Could you check a few things on this model? Use its own coordinates, in mm. Coordinates: 2 decimals unless noted, no trailing zeros. Loops run counter-clockwise (first coordinate to the right, second up) from the corner with the lowest first, then second, coordinate; pieces in that order, holes last. Notation, with made-up numbers: (73.25, -24) - (93.25, -24) arc R30 ccw to (93.25, 9) - close; hole circle Ø9 at (84, 79.5). An arc over 180 degrees is marked (long way). One line per item, written item: value. Start each with the question number.
(1) I'm going to push flat-ended pins straight in: P1, Ø2, axis at x = -120.5, z = 3, coming from the -Y side; P2, Ø1.5, axis at x = -78.5, y = 12.5, coming from the -Z side; P3, Ø3.5, axis at x = -36, z = 1.5, coming from the -Y side; P4, Ø2.5, axis at x = -160.43, y = -41.87, coming from the -Z side. Where does each tip first touch, or does it pass through?
(2) If I drill on line 1 along Y through (x, z) = (-158, 2.5); line 2 along Y through (x, z) = (-161, 4.25); line 3 along Y through (x, z) = (-144, 1.75), over which ranges is the centre line in solid material (lowest first)? Write a range as from..to.
(3) If we section it at B-B on x = -134: Write out the boundary of the cut face in (y, z), then the cut area to 3 significant figures.
(4) If we section it at C-C on x = -38: Count the separate pieces of the cut face and the enclosed holes in it, then the cut area to 3 significant figures.
(5) If we section it at A-A on z = -1: Write out the boundary of the cut face in (x, y), then the cut area to 3 significant figures.
```python
from build123d import *

# Parameters (mm, degrees)
F0_R     = 1.5
F0_R_2   = 4.064442
F0_W     = 17.869964
F0_H     = 3
F1_DEPTH = 4.5
F2_W     = 10.996489
F2_H     = 3.251471
F3_DEPTH = 2
F4_R     = 5.902111
F5_DEPTH = 2
F7_DEPTH = 25


with BuildPart() as f1:
    # F0 (on Top) → F1 (new body)
    with BuildSketch(Plane.XY):
        with BuildLine():
            ThreePointArc((0, 42.5), (-1.464466, 46.035534), (-5, 47.5))
            Line((-5, 47.5), (-22.221084, 47.5))
            ThreePointArc((-22.221084, 47.5), (-23.18507, 47.406193), (-24.112885, 47.128292))
            Line((-24.112885, 47.128292), (-53.784762, 35))
            Line((-53.784762, 35), (-94.883973, 35))
            ThreePointArc((-94.883973, 35), (-97.317732, 34.367701), (-99.135947, 32.630726))
            ThreePointArc((-99.135947, 32.630726), (-115.303652, 25.021468), (-128.810321, 36.720415))
            ThreePointArc((-128.810321, 36.720415), (-129.96409, 38.753765), (-131.916134, 40.040317))
            Line((-131.916134, 40.040317), (-152.559489, 47.5))
            Line((-152.559489, 47.5), (-165, 47.5))
            ThreePointArc((-165, 47.5), (-168.535534, 46.035534), (-170, 42.5))
            Line((-170, 42.5), (-170, 35))
            Line((-170, 35), (-170, 0))
            Line((-170, 0), (-170, -35))
            Line((-170, -35), (-170, -42.5))
            ThreePointArc((-170, -42.5), (-168.535534, -46.035534), (-165, -47.5))
            Line((-165, -47.5), (-152.559489, -47.5))
            Line((-152.559489, -47.5), (-131.916134, -40.040317))
            ThreePointArc((-131.916134, -40.040317), (-129.96409, -38.753765), (-128.810321, -36.720415))
            ThreePointArc((-128.810321, -36.720415), (-115.303652, -25.021468), (-99.135947, -32.630726))
            ThreePointArc((-99.135947, -32.630726), (-97.317732, -34.367701), (-94.883973, -35))
            Line((-94.883973, -35), (-53.784762, -35))
            Line((-53.784762, -35), (-24.112885, -47.128292))
            ThreePointArc((-24.112885, -47.128292), (-23.18507, -47.406193), (-22.221084, -47.5))
            Line((-22.221084, -47.5), (-5, -47.5))
            ThreePointArc((-5, -47.5), (-1.464466, -46.035534), (0, -42.5))
            Line((0, -42.5), (0, -35))
            Line((0, -35), (0, 0))
            Line((0, 0), (0, 35))
            Line((0, 35), (0, 42.5))
        make_face()
        with Locations((-160.42681, -41.874927)):
            Circle(F0_R, mode=Mode.SUBTRACT)
        with Locations((-165.596247, -31.161871)):
            Circle(F0_R, mode=Mode.SUBTRACT)
        with Locations((-157.563224, -27.604574)):
            Circle(F0_R_2, mode=Mode.SUBTRACT)
        with Locations((-94.883973, -30)):
            Circle(F0_R, mode=Mode.SUBTRACT)
        with BuildLine():
            Line((-155.63046, -13.178692), (-144.869025, -2.417256))
            ThreePointArc((-144.869025, -2.417256), (-142.747705, -2.417256), (-142.747705, -4.538577))
            Line((-142.747705, -4.538577), (-153.50914, -15.300012))
            ThreePointArc((-153.50914, -15.300012), (-155.63046, -15.300012), (-155.63046, -13.178692))
        make_face(mode=Mode.SUBTRACT)
        with BuildLine():
            Line((-126.950468, -15.501301), (-137.913192, -4.538577))
            ThreePointArc((-137.913192, -4.538577), (-137.913192, -2.417256), (-135.791872, -2.417256))
            Line((-135.791872, -2.417256), (-124.829148, -13.37998))
            ThreePointArc((-124.829148, -13.37998), (-124.829148, -15.501301), (-126.950468, -15.501301))
        make_face(mode=Mode.SUBTRACT)
        with Locations((-97.036146, -19.152308)):
            Circle(F0_R_2, mode=Mode.SUBTRACT)
        with Locations((-11.601751, -41.25)):
            Circle(F0_R, mode=Mode.SUBTRACT)
        with Locations((-37.462216, -31.5)):
            Rectangle(F0_W, F0_H, mode=Mode.SUBTRACT)
        with Locations((-3.568025, -34.615397)):
            Circle(F0_R, mode=Mode.SUBTRACT)
        with BuildLine():
            ThreePointArc((-155.63046, 13.178692), (-155.63046, 15.300012), (-153.50914, 15.300012))
            Line((-153.50914, 15.300012), (-142.747705, 4.538577))
            ThreePointArc((-142.747705, 4.538577), (-142.747705, 2.417256), (-144.869025, 2.417256))
            Line((-144.869025, 2.417256), (-155.63046, 13.178692))
        make_face(mode=Mode.SUBTRACT)
        with BuildLine():
            ThreePointArc((-135.791872, 2.417256), (-137.913192, 2.417256), (-137.913192, 4.538577))
            Line((-137.913192, 4.538577), (-126.950468, 15.501301))
            ThreePointArc((-126.950468, 15.501301), (-124.829148, 15.501301), (-124.829148, 13.37998))
            Line((-124.829148, 13.37998), (-135.791872, 2.417256))
        make_face(mode=Mode.SUBTRACT)
        with Locations((-97.036146, 19.152308)):
            Circle(F0_R_2, mode=Mode.SUBTRACT)
        with Locations((-157.563224, 27.604574)):
            Circle(F0_R_2, mode=Mode.SUBTRACT)
        with Locations((-165.596247, 31.161871)):
            Circle(F0_R, mode=Mode.SUBTRACT)
        with Locations((-160.42681, 41.874927)):
            Circle(F0_R, mode=Mode.SUBTRACT)
        with Locations((-94.883973, 30)):
            Circle(F0_R, mode=Mode.SUBTRACT)
        with Locations((-37.462216, 31.5)):
            Rectangle(F0_W, F0_H, mode=Mode.SUBTRACT)
        with Locations((-3.568025, 34.615397)):
            Circle(F0_R, mode=Mode.SUBTRACT)
        with Locations((-11.601751, 41.25)):
            Circle(F0_R, mode=Mode.SUBTRACT)
    extrude(amount=F1_DEPTH)

    # F2 (on face) → F3 (join)
    with BuildSketch(Plane(origin=(0, 0, 0), x_dir=(1, 0, 0), z_dir=(0, 0, -1))):
        with Locations((-164.501756, 34.962811)):
            Rectangle(F2_W, F2_H)
        with BuildLine():
            Line((-0.535832, 44.751933), (-7.695868, 37.591897))
            Line((-7.695868, 37.591897), (-5.774221, 35.670251))
            Line((-5.774221, 35.670251), (0, 40.31283))
            Line((0, 40.31283), (0, 42.5))
            ThreePointArc((0, 42.5), (-0.135802, 43.657402), (-0.535832, 44.751933))
        make_face()
        with BuildLine():
            Line((0, -42.5), (0, -40.31283))
            Line((0, -40.31283), (-5.774221, -35.670251))
            Line((-5.774221, -35.670251), (-7.695868, -37.591897))
            Line((-7.695868, -37.591897), (-0.535832, -44.751933))
            ThreePointArc((-0.535832, -44.751933), (-0.135802, -43.657402), (0, -42.5))
        make_face()
        with Locations((-164.501756, -34.962811)):
            Rectangle(F2_W, F2_H)
    extrude(amount=F3_DEPTH)

    # F4 (on face) → F5 (cut)
    with BuildSketch(Plane(origin=(0, 0, 0), x_dir=(1, 0, 0), z_dir=(0, 0, -1))):
        with Locations((-97.036146, 19.152308)):
            Circle(F4_R)
        with Locations((-157.563224, 27.604574)):
            Circle(F4_R)
        with Locations((-97.036146, -19.152308)):
            Circle(F4_R)
        with Locations((-157.563224, -27.604574)):
            Circle(F4_R)
    extrude(amount=-F5_DEPTH, mode=Mode.SUBTRACT)

    # F6 (on face) → F7 (cut)
    with BuildSketch(Plane(origin=(0, 0, 0), x_dir=(1, 0, 0), z_dir=(0, 0, -1))):
        with BuildLine():
            ThreePointArc((-79.22934, 23.110536), (-80.72934, 21.610536), (-79.22934, 20.110536))
            Line((-79.22934, 20.110536), (-20.462809, 20.110536))
            ThreePointArc((-20.462809, 20.110536), (-18.962809, 21.610536), (-20.462809, 23.110536))
            Line((-20.462809, 23.110536), (-79.22934, 23.110536))
        make_face()
        with BuildLine():
            Line((-20.462809, 18.110536), (-79.22934, 18.110536))
            ThreePointArc((-79.22934, 18.110536), (-80.72934, 16.610536), (-79.22934, 15.110536))
            Line((-79.22934, 15.110536), (-20.462809, 15.110536))
            ThreePointArc((-20.462809, 15.110536), (-18.962809, 16.610536), (-20.462809, 18.110536))
        make_face()
        with BuildLine():
            Line((-20.462809, 13.110536), (-79.22934, 13.110536))
            ThreePointArc((-79.22934, 13.110536), (-80.72934, 11.610536), (-79.22934, 10.110536))
            Line((-79.22934, 10.110536), (-20.462809, 10.110536))
            ThreePointArc((-20.462809, 10.110536), (-18.962809, 11.610536), (-20.462809, 13.110536))
        make_face()
        with BuildLine():
            Line((-20.462809, 8.110536), (-79.22934, 8.110536))
            ThreePointArc((-79.22934, 8.110536), (-80.72934, 6.610536), (-79.22934, 5.110536))
            Line((-79.22934, 5.110536), (-20.462809, 5.110536))
            ThreePointArc((-20.462809, 5.110536), (-18.962809, 6.610536), (-20.462809, 8.110536))
        make_face()
        with BuildLine():
            Line((-20.462809, 3.110536), (-79.22934, 3.110536))
            ThreePointArc((-79.22934, 3.110536), (-80.72934, 1.610536), (-79.22934, 0.110536))
            Line((-79.22934, 0.110536), (-20.462809, 0.110536))
            ThreePointArc((-20.462809, 0.110536), (-18.962809, 1.610536), (-20.462809, 3.110536))
        make_face()
        with BuildLine():
            Line((-20.462809, -1.889464), (-79.22934, -1.889464))
            ThreePointArc((-79.22934, -1.889464), (-80.72934, -3.389464), (-79.22934, -4.889464))
            Line((-79.22934, -4.889464), (-20.462809, -4.889464))
            ThreePointArc((-20.462809, -4.889464), (-18.962809, -3.389464), (-20.462809, -1.889464))
        make_face()
        with BuildLine():
            Line((-20.462809, -6.889464), (-79.22934, -6.889464))
            ThreePointArc((-79.22934, -6.889464), (-80.72934, -8.389464), (-79.22934, -9.889464))
            Line((-79.22934, -9.889464), (-20.462809, -9.889464))
            ThreePointArc((-20.462809, -9.889464), (-18.962809, -8.389464), (-20.462809, -6.889464))
        make_face()
        with BuildLine():
            Line((-20.462809, -11.889464), (-79.22934, -11.889464))
            ThreePointArc((-79.22934, -11.889464), (-80.72934, -13.389464), (-79.22934, -14.889464))
            Line((-79.22934, -14.889464), (-20.462809, -14.889464))
            ThreePointArc((-20.462809, -14.889464), (-18.962809, -13.389464), (-20.462809, -11.889464))
        make_face()
        with BuildLine():
            Line((-20.462809, -16.889464), (-79.22934, -16.889464))
            ThreePointArc((-79.22934, -16.889464), (-80.72934, -18.389464), (-79.22934, -19.889464))
            Line((-79.22934, -19.889464), (-20.462809, -19.889464))
            ThreePointArc((-20.462809, -19.889464), (-18.962809, -18.389464), (-20.462809, -16.889464))
        make_face()
        with BuildLine():
            Line((-20.462809, -21.889464), (-79.22934, -21.889464))
            ThreePointArc((-79.22934, -21.889464), (-80.72934, -23.389464), (-79.22934, -24.889464))
            Line((-79.22934, -24.889464), (-20.462809, -24.889464))
            ThreePointArc((-20.462809, -24.889464), (-18.962809, -23.389464), (-20.462809, -21.889464))
        make_face()
    extrude(amount=-F7_DEPTH, mode=Mode.SUBTRACT)


solid = f1.part
```
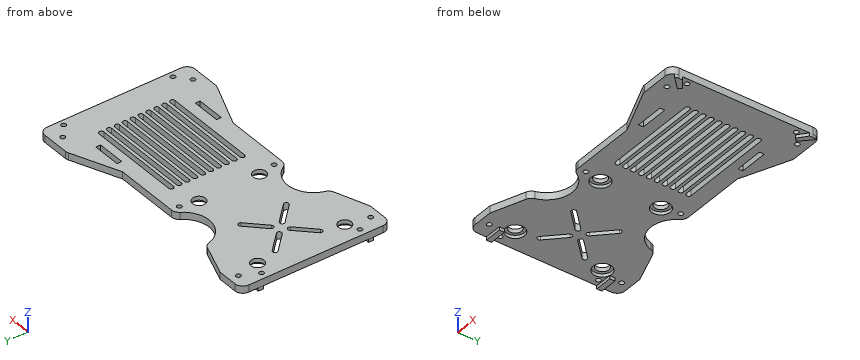
Values:
1. P1: stops at y = -27.21
1. P2: stops at z = 0
1. P3: stops at y = -42.98
1. P4: passes through
2. line 1: y = -47.5..-31.65, -23.56..23.56, 31.65..47.5
2. line 2: y = -47.5..-43.26, -40.49..-29.77, -25.43..25.43, 29.77..40.49, 43.26..47.5
2. line 3: y = -44.41..-5.79, -1.99..1.99, 5.79..44.41
3. outline: (-40.79, 0) - (-8.45, 0) - (-8.45, 4.5) - (-40.79, 4.5) - close; (-4.21, 0) - (4.21, 0) - (4.21, 4.5) - (-4.21, 4.5) - close; (8.45, 0) - (40.79, 0) - (40.79, 4.5) - (8.45, 4.5) - close
3. area: 329 mm2
4. separate pieces: 13
4. enclosed holes: 0
4. area: 211 mm2
5. outline: (-170, -36.59) - (-159, -36.59) - (-159, -33.34) - (-170, -33.34) - close; (-170, 33.34) - (-159, 33.34) - (-159, 36.59) - (-170, 36.59) - close; (-7.7, -37.59) - (-0.54, -44.75) arc R5 ccw to (0, -42.5) - (0, -40.31) - (-5.77, -35.67) - close; (-7.7, 37.59) - (-5.77, 35.67) - (0, 40.31) - (0, 42.5) arc R5 ccw to (-0.54, 44.75) - close
5. area: 129 mm2
